```python
from build123d import *

# Parameters (mm, degrees)
BOSS_EXTRUDE1_DEPTH  = 20
SKETCH2_W            = 5
SKETCH2_H            = 20
BOSS_EXTRUDE2_DEPTH  = 5
CUT_EXTRUDE1_DEPTH   = 5
SKETCH4_W            = 5
SKETCH4_H            = 10
BOSS_EXTRUDE3_DEPTH  = 5
CUT_EXTRUDE2_DEPTH   = 5
BOSS_EXTRUDE31_DEPTH = 20
CUT_EXTRUDE11_DEPTH  = 25
SKETCH24_W           = 5
SKETCH24_H           = 15
BOSS_EXTRUDE32_DEPTH = 5
CUT_EXTRUDE12_DEPTH  = 5
BOSS_EXTRUDE33_DEPTH = 5
BOSS_EXTRUDE34_DEPTH = 5


with BuildPart() as part:
    # Sketch1 → Boss-Extrude1 (new body)
    with BuildSketch(Plane(origin=(0, 0, 0), x_dir=(1, 0, 0), z_dir=(0, 1, 0))):
        Polygon((-15, 0), (0, 0), (0, -15), (-5, -15), (-5, -10), align=None)
    extrude(amount=-BOSS_EXTRUDE1_DEPTH)

    # Sketch2 → Boss-Extrude2 (add)
    with BuildSketch(Plane.XY.offset(15)):
        with Locations((-2.5, -10)):
            Rectangle(SKETCH2_W, SKETCH2_H)
    extrude(amount=BOSS_EXTRUDE2_DEPTH)

    # Sketch3 → Cut-Extrude1 (cut)
    with BuildSketch(Plane.ZY.offset(5)):
        Polygon((15, 0), (20, -5), (20, 0), align=None)
    extrude(amount=-CUT_EXTRUDE1_DEPTH, mode=Mode.SUBTRACT)

    # Sketch4 → Boss-Extrude3 (add)
    with BuildSketch(Plane.ZY.offset(5)):
        with Locations((17.5, -15)):
            Rectangle(SKETCH4_W, SKETCH4_H)
    extrude(amount=BOSS_EXTRUDE3_DEPTH)

    # Sketch5 → Cut-Extrude2 (cut)
    with BuildSketch(Plane.XY.offset(20)):
        Polygon((-5, -10), (-10, -15), (-10, -10), align=None)
    extrude(amount=-CUT_EXTRUDE2_DEPTH, mode=Mode.SUBTRACT)

    # Sketch14 → Boss-Extrude31 (add)
    with BuildSketch(Plane(origin=(0, -20, 0), x_dir=(-1, 0, 0), z_dir=(0, -1, 0))):
        Polygon((15, 0), (5, -10), (5, -15), (10, -15), (15, -10), align=None)
    extrude(amount=-BOSS_EXTRUDE31_DEPTH)

    # 3DSketch7 → Cut-Extrude11 (cut, along a direction that is not the sketch's normal)
    with BuildSketch(Plane(origin=(-15, 0, 0), x_dir=(0.5345224838248488, -0.2672612419124244, 0.8017837257372732), z_dir=(0.5773502691896258, -0.5773502691896258, -0.5773502691896258))):
        Polygon((0, 0), (13.363062096, -4.629100499), (18.708286934, 0), (17.371980724, 6.943650748), (10.690449676, 9.258200998), align=None)
    extrude(amount=-CUT_EXTRUDE11_DEPTH, dir=(0, 0, -1), mode=Mode.SUBTRACT)

    # Sketch24 → Boss-Extrude32 (add)
    with BuildSketch(Plane.ZY.offset(15)):
        with Locations((2.5, -12.5)):
            Rectangle(SKETCH24_W, SKETCH24_H)
    extrude(amount=BOSS_EXTRUDE32_DEPTH)

    # Sketch25 → Cut-Extrude12 (cut)
    with BuildSketch(Plane.XY.offset(5)):
        Polygon((-15, -5), (-20, -5), (-20, -10), align=None)
    extrude(amount=-CUT_EXTRUDE12_DEPTH, mode=Mode.SUBTRACT)

    # Sketch26 → Boss-Extrude33 (add)
    with BuildSketch(Plane(origin=(0, -20, 0), x_dir=(-1, 0, 0), z_dir=(0, -1, 0))):
        Polygon((20, -5), (15, -5), (15, -10), (10, -15), (15, -15), (20, -10), align=None)
    extrude(amount=-BOSS_EXTRUDE33_DEPTH)

    # Sketch27 → Boss-Extrude34 (add)
    with BuildSketch(Plane(origin=(0, -15, 0), x_dir=(1, 0, 0), z_dir=(0, 1, 0))):
        Polygon((-20, -5), (-15, -5), (-15, -10), align=None)
    extrude(amount=BOSS_EXTRUDE34_DEPTH)


solid = part.part
```
The model under review builds one solid part; all positions refer to its coordinate system, in mm. A direction names the side the tool comes from. Give positions to 0.01 mm unless a question says otherwise; leave off trailing zeros. Write each loop counter-clockwise with the first axis right and the second up, starting at its lowest first coordinate (ties: lowest second). Pieces come first, ordered by that corner, then holes. Notation, with made-up numbers: (26.5, -36.5) -> (32.5, -36.5) arc R7 ccw to (32.5, -29.5) -> close; hole circle Ø1 at (35, -14.5). An arc over 180 degrees is marked (long way). Put each result on its own line as item: value.
(1) We need section A-A, the plane x = -16. Give the boundary of the cut face in (y, z), and give its area (3 significant figures).
Results are:
outline: (-20, 0) -> (-6, 0) -> (-6, 5) -> (-10, 5) -> (-10, 9) -> (-15, 9) -> (-15, 14) -> (-20, 14) -> close
area: 135 mm²
(2) The part is to be moulded in two halves that separate along Y. For faces 1 (the flat face through (-10, -10, 0)), 2 (the flat face through (-17, -10, 7)), say which applies: pulls with the +Y half, pulls with the -Y half, needs draft (parallel to the pull), parting line crosses it, or undercut.
Results are:
face 1: needs draft
face 2: pulls with the +Y half
(3) To check wall thickness, follow probe 1 along Z at (x, y) = (-5.25, -10); probe 2 along X at (y, z) = (-4.5, 3.75); probe 3 along X at (y, z) = (-1.25, 5.5). State the ranges of each line that lie inside material, in increasing order. Write a range as from..to.
Results are:
probe 1: 0..15
probe 2: -15..0
probe 3: -10.75..0
(4) We need section B-B, the plane y = -15.5. Give the boundary of the cut face in (x, z), and give its area (4 significant figures).
Results are:
outline: (-20, 0) -> (0, 0) -> (0, 20) -> (-10, 20) -> (-10, 15) -> (-15, 15) -> (-20, 10) -> close
area: 337.5 mm²
(5) We need section D-D, the plane x = -6.25. Give the boundary of the cut face in (y, z), and give its area (3 significant figures).
Results are:
outline: (-20, 0) -> (0, 0) -> (0, 8.75) -> (-6.25, 15) -> (-11.25, 15) -> (-11.25, 20) -> (-20, 20) -> close
area: 324 mm²
(6) For pin 1 Ø5.5 at (y, z) = (-17.5, 17.5) entering from -X; pin 2 Ø1.5 at (y, z) = (-3, 2.5) entering from -X; pin 3 Ø3 at (y, z) = (-13.5, 11.5) entering from +X; pin 4 Ø4 at (x, y) = (-16.5, -8) entering from +Z, all flat-tipped, find the tip position at first contact; note any pin that passes through.
Results are:
pin 1: x = -15.25
pin 2: x = -15
pin 3: x = 0
pin 4: z = 9.32
(7) Tool access review of faces 3 (the flat face through (-15, -4, 1)), 4 (the flat face through (-12, -18, 15)), 5 (the flat face through (-15, -9, 6)): name each direction out of +Z, -Z, +X, -X, +Y, -Y from which nothing blocks a thin tool from reaching the whole face with its end or side.
Results are:
face 3: +Z, -Z, -X, +Y
face 4: +Z, -X, +Y, -Y
face 5: +Z, -X, +Y
(8) We need section C-C, the plane z = 5.5. Give the boundary of the cut face in (x, y).
Results are:
outline: (-20, -20) -> (0, -20) -> (0, 0) -> (-9.5, 0) -> (-15, -5.5) -> (-15, -10) -> (-19.5, -10) -> (-19.5, -15) -> (-20, -15) -> close
